Input: dimensioned drawing with shaded views. Units: mm. Origin: part minimum x, y, z. A direction names the side the tool comes from. Give positions to 0.01 mm unless a question says otherwise; leave off trailing zeros. Write each loop counter-clockwise with the first axis right and the second up, starting at its lowest first coordinate (ties: lowest second). Pieces come first, ordered by that corner, then holes.
Q1. Pin query (flat end, axial travel): pin 1 Ø2.5 at (x, z) = (1, 33) entering from -Y; pin 2 Ø4 at (x, y) = (39.5, 15) entering from -Z. Return the tip coordinate at first contact, or that it passes through.
Q2. Mould query, pull axis X, two halves, no side actions, for the marked faces 1, 2 and 3. Classes: +X half, -X half, draft (parallel to the pull), parting line (faces both ways), or undercut.
Q3. Section B-B (z = 4). Return the cut outline in (x, y).
Q4. Section D-D (y = 18). Return the cut outline in (x, z), plus the area to 3 significant figures.
Q5. Line query: line 1 (Y direction, x = 14.5, z = 47.35); line 2 (X direction, y = 45.5, z = 28); line 3 (Z direction, x = 34.5, y = 7.5). Output: solid intervals per line, ascending.
Q6. Reachability of the marked faces 4 and 5 from +Z, -Z, +X, -X, +Y, -Y: full face, straight path, thin tool, end or side. Return the list, or none.
Q7. Section C-C (x = 39.5). Return the cut outline in (y, z), plus the area to 4 significant figures.
Q8. Section A-A (y = 5). Return the cut outline in (x, z), plus the area to 3 significant figures.
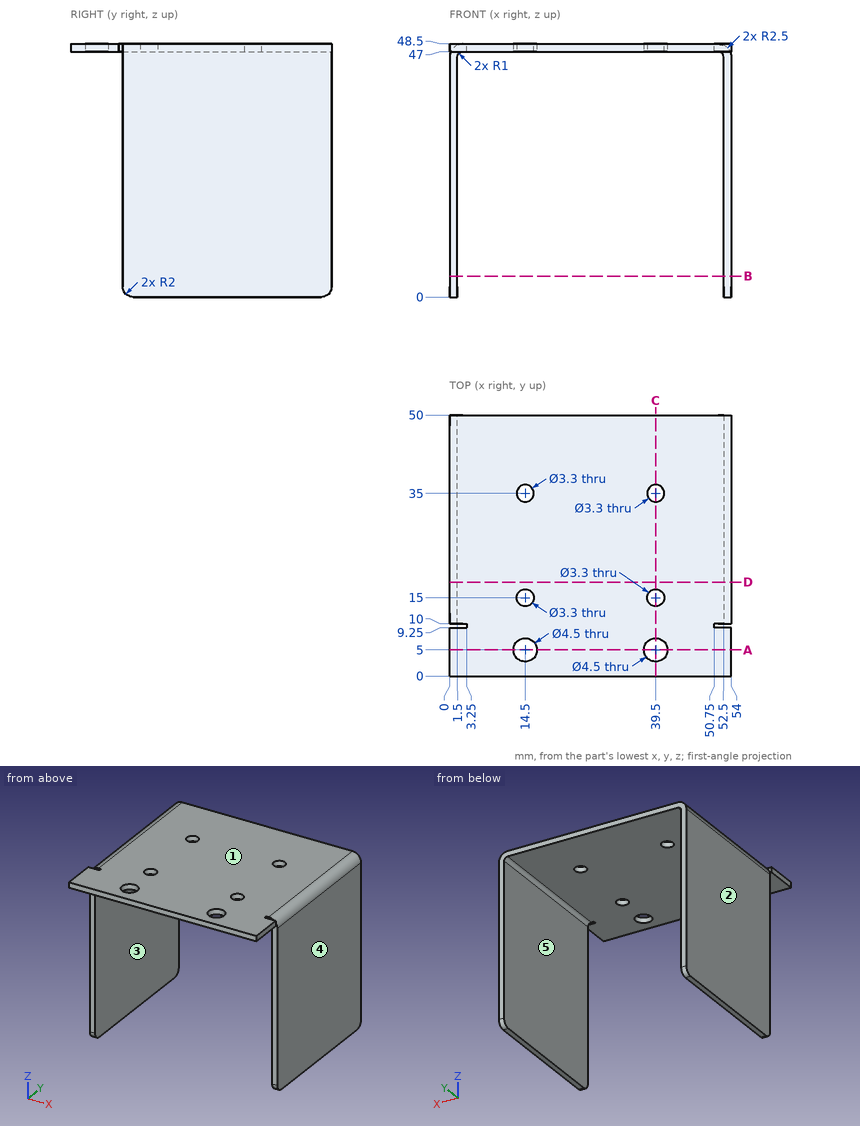
Computed:
1. pin 1: stops at y = 10
1. pin 2: stops at z = 47
2. face 1: draft
2. face 2: -X half
2. face 3: undercut
3. outline: (0, 10) - (1.5, 10) - (1.5, 50) - (0, 50) - close; (52.5, 10) - (54, 10) - (54, 50) - (52.5, 50) - close
4. outline: (0, 0) - (1.5, 0) - (1.5, 46) arc R1 cw to (2.5, 47) - (51.5, 47) arc R1 cw to (52.5, 46) - (52.5, 0) - (54, 0) - (54, 46) arc R2.5 ccw to (51.5, 48.5) - (2.5, 48.5) arc R2.5 ccw to (0, 46) - close
4. area: 220 mm2
5. line 1: y = 0 to 2.75, 7.25 to 13.35, 16.65 to 33.35, 36.65 to 50
5. line 2: x = 0 to 1.5, 52.5 to 54
5. line 3: z = 47 to 48.5
6. face 4: +Z, -Z, +X, +Y, -Y
6. face 5: -Z, +Y, -Y
7. outline: (0, 47) - (2.75, 47) - (2.75, 48.5) - (0, 48.5) - close; (7.25, 47) - (13.35, 47) - (13.35, 48.5) - (7.25, 48.5) - close; (16.65, 47) - (33.35, 47) - (33.35, 48.5) - (16.65, 48.5) - close; (36.65, 47) - (50, 47) - (50, 48.5) - (36.65, 48.5) - close
7. area: 58.35 mm2
8. outline: (0, 47) - (12.25, 47) - (12.25, 48.5) - (0, 48.5) - close; (16.75, 47) - (37.25, 47) - (37.25, 48.5) - (16.75, 48.5) - close; (41.75, 47) - (54, 47) - (54, 48.5) - (41.75, 48.5) - close
8. area: 67.5 mm2
